Answer from the drawing. Dimensions are ordinates in mm from the lowest x, y and z of the part. A direction names the side the tool comes from. Give positions to 0.01 mm unless a question says otherwise; leave off trailing zeros. Loops run counter-clockwise (first coordinate to the right, second up) from the corner with the lowest first, then second, coordinate; pieces in that order, holes last.
Item 1: Consider line 1 along Y through (x, z) = (9.12, 7); line 2 along Z through (x, y) = (8.5, 2.25). Determine where each line is inside the solid, lowest interval first.
Item 2: A tool of negligible diameter and unlimited length cuts with its end or side. For the marked faces 4 and 5, from which of +Z, -Z, +X, -X, +Y, -Y can it reach the whole face along a straight path? Write none if from no direction.
Item 3: Section C-C, the plane z = 10.5 is taken. Give the vertices of the cut face in (x, y).
Item 4: Each of these flat-tipped pins is pushed along its axis until it touches: pin 1 Ø3 at (x, z) = (2.5, 18) entering from +Y; pin 2 Ø5 at (x, z) = (13, 9.5) entering from -Y (3 decimals); pin 3 Ø2 at (y, z) = (17.5, 19.5) entering from +X; pin 4 Ø1.2 at (x, y) = (8.5, 1) entering from +Z. Where does it stop, or does it pass through?
Item 5: Section A-A, the plane x = 9.12 is taken. Give the vertices of the cut face in (y, z), and give its area (3 significant figures).
Item 6: The mould has two halves that part along X. Classify the marked faces 1, 2 and 3: pulls with the +X half, pulls with the -X half, needs draft (parallel to the pull), parting line crosses it, or undercut.
Item 7: Section B-B, the plane y = 9.12 is taken. Give the vertices of the cut face in (x, z).
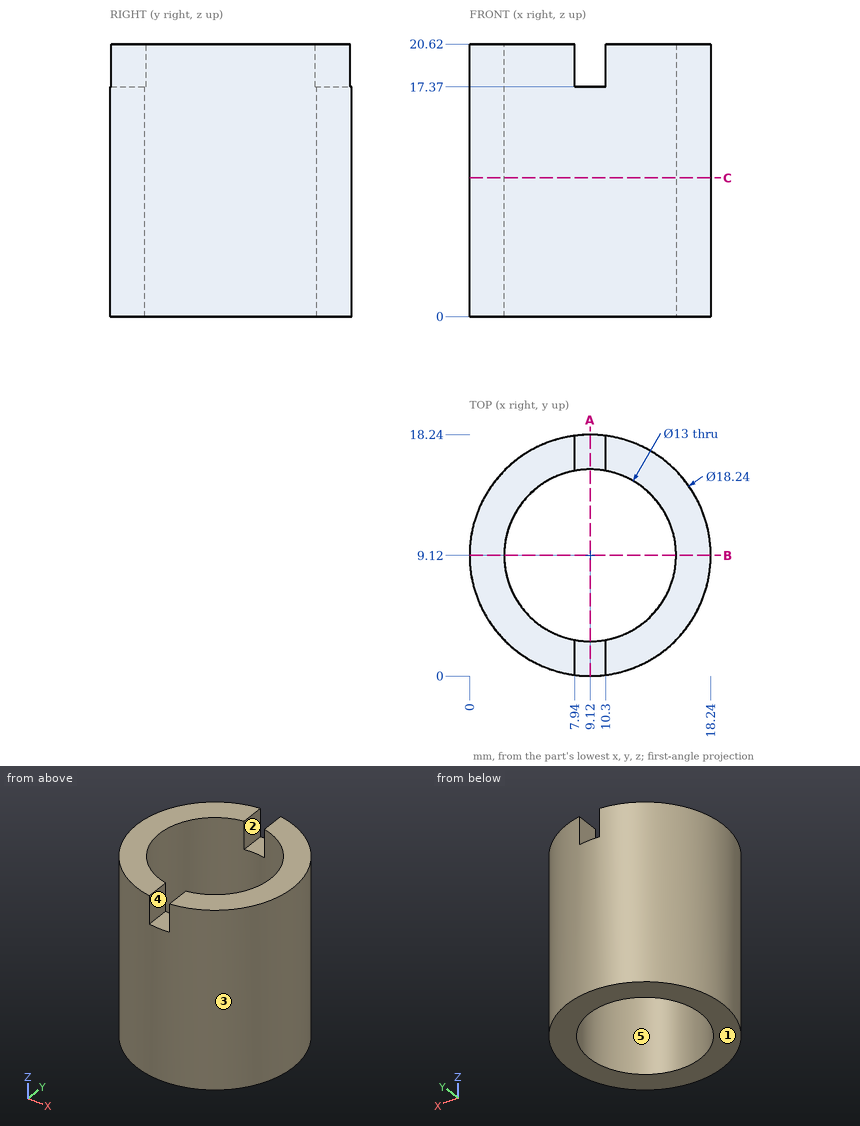
Worked answers:
1. line 1: y = 0 to 2.62, 15.62 to 18.24
1. line 2: z = 0 to 17.37
2. face 4: +Z, +Y, -Y
2. face 5: +Z, -Z
3. outline: circle Ø18.24 at (9.12, 9.12); hole circle Ø13 at (9.12, 9.12)
4. pin 1: stops at y = 16.67
4. pin 2: stops at y = 0.105
4. pin 3: stops at x = 14.48
4. pin 4: stops at z = 20.62
5. outline: (0, 0) - (2.62, 0) - (2.62, 17.37) - (0, 17.37) - close; (15.62, 0) - (18.24, 0) - (18.24, 17.37) - (15.62, 17.37) - close
5. area: 91.0 mm2
6. face 1: needs draft
6. face 2: undercut
6. face 3: parting line crosses it
7. outline: (0, 0) - (2.62, 0) - (2.62, 20.62) - (0, 20.62) - close; (15.62, 0) - (18.24, 0) - (18.24, 20.62) - (15.62, 20.62) - close
